```python
from build123d import *

# Parameters (mm, degrees)
SKETCH3_R            = 12.7
BOSS_EXTRUDE1_DEPTH  = 76.2
BOSS_EXTRUDE2_DEPTH  = 6.35
SKETCH6_W            = 63.5
SKETCH6_H            = 50.8
BOSS_EXTRUDE3_DEPTH  = 6.35
SKETCH9_W            = 50.8
SKETCH9_H            = 6.35
BOSS_EXTRUDE4_DEPTH  = 0.38862
SKETCH10_W           = 0.38862
SKETCH10_H           = 50.8
BOSS_EXTRUDE5_DEPTH  = 25.4
SKETCH11_W           = 50.8
SKETCH11_H           = 6.35
BOSS_EXTRUDE6_DEPTH  = 0.38862
SKETCH13_W           = 0.38862
SKETCH13_H           = 50.8
BOSS_EXTRUDE7_DEPTH  = 25.4
SKETCH14_W           = 0.38862
SKETCH14_H           = 50.8
BOSS_EXTRUDE8_DEPTH  = 10.8712
SKETCH15_W           = 50.8
SKETCH15_H           = 10.8712
BOSS_EXTRUDE9_DEPTH  = 25.76322
SKETCH16_W           = 0.38862
SKETCH16_H           = 50.8
BOSS_EXTRUDE10_DEPTH = 10.8712
SKETCH17_W           = 50.8
SKETCH17_H           = 10.8712
BOSS_EXTRUDE11_DEPTH = 25.76322


with BuildPart() as part:
    # Sketch3 → Boss-Extrude1 (new body)
    with BuildSketch(Plane.XY):
        with Locations(Location((0, 0, 0), (0, 0, 180))):
            Circle(SKETCH3_R)
    extrude(amount=BOSS_EXTRUDE1_DEPTH)

    # Sketch4 → Boss-Extrude2 (add)
    with BuildSketch(Plane(origin=(0, 0, 0), x_dir=(-1, 0, 0), z_dir=(0, 0, -1))):
        Polygon((0, 0), (19.05, 0), (19.05, 50.8), (-19.05, 50.8), (-19.05, 0), align=None)
    extrude(amount=-BOSS_EXTRUDE2_DEPTH)

    # Sketch6 → Boss-Extrude3 (add)
    with BuildSketch(Plane(origin=(0, 50.8, 0), x_dir=(1, 0, 0), z_dir=(0, 1, 0))):
        with Locations((1.04805825, -17.613482739)):
            Rectangle(SKETCH6_W, SKETCH6_H)
    extrude(amount=BOSS_EXTRUDE3_DEPTH)

    # Sketch9 → Boss-Extrude4 (add)
    with BuildSketch(Plane(origin=(32.79805825, 0, 0), x_dir=(0, 0, -1), z_dir=(1, 0, 0))):
        with Locations((-17.613482739, 53.975)):
            Rectangle(SKETCH9_W, SKETCH9_H)
    extrude(amount=BOSS_EXTRUDE4_DEPTH)

    # Sketch10 → Boss-Extrude5 (add)
    with BuildSketch(Plane(origin=(0, 57.15, 0), x_dir=(1, 0, 0), z_dir=(0, 1, 0))):
        with Locations((32.99236825, -17.613482739)):
            Rectangle(SKETCH10_W, SKETCH10_H)
    extrude(amount=BOSS_EXTRUDE5_DEPTH)

    # Sketch11 → Boss-Extrude6 (add)
    with BuildSketch(Plane.ZY.offset(30.70194175)):
        with Locations((17.613482739, 53.975)):
            Rectangle(SKETCH11_W, SKETCH11_H)
    extrude(amount=BOSS_EXTRUDE6_DEPTH)

    # Sketch13 → Boss-Extrude7 (add)
    with BuildSketch(Plane(origin=(0, 57.15, 0), x_dir=(1, 0, 0), z_dir=(0, 1, 0))):
        with Locations((-30.89625175, -17.613482739)):
            Rectangle(SKETCH13_W, SKETCH13_H)
    extrude(amount=BOSS_EXTRUDE7_DEPTH)

    # Sketch14 → Boss-Extrude8 (add)
    with BuildSketch(Plane(origin=(0, 82.55, 0), x_dir=(1, 0, 0), z_dir=(0, 1, 0))):
        with Locations((-30.89625175, -17.613482739)):
            Rectangle(SKETCH14_W, SKETCH14_H)
    extrude(amount=BOSS_EXTRUDE8_DEPTH)

    # Sketch15 → Boss-Extrude9 (add)
    with BuildSketch(Plane(origin=(-30.70194175, 0, 0), x_dir=(0, 0, -1), z_dir=(1, 0, 0))):
        with Locations((-17.613482739, 87.9856)):
            Rectangle(SKETCH15_W, SKETCH15_H)
    extrude(amount=BOSS_EXTRUDE9_DEPTH)

    # Sketch16 → Boss-Extrude10 (add)
    with BuildSketch(Plane(origin=(0, 82.55, 0), x_dir=(1, 0, 0), z_dir=(0, 1, 0))):
        with Locations((32.99236825, -17.613482739)):
            Rectangle(SKETCH16_W, SKETCH16_H)
    extrude(amount=BOSS_EXTRUDE10_DEPTH)

    # Sketch17 → Boss-Extrude11 (add)
    with BuildSketch(Plane.ZY.offset(-32.79805825)):
        with Locations((17.613482739, 87.9856)):
            Rectangle(SKETCH17_W, SKETCH17_H)
    extrude(amount=BOSS_EXTRUDE11_DEPTH)


solid = part.part
```
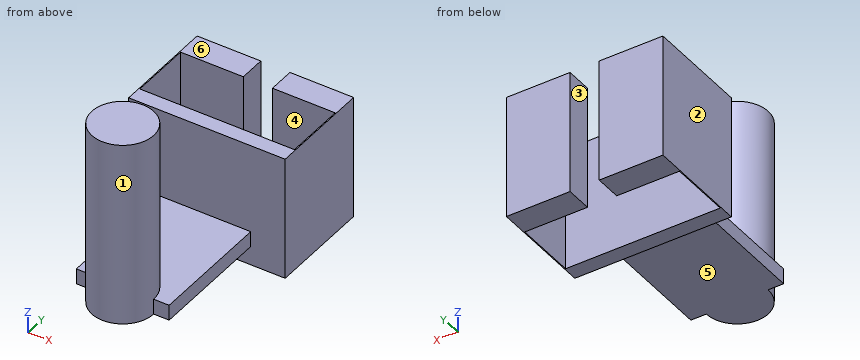
Geometry check sheet. Reference: the model listing, model coordinates, mm. Face numbers are marked on the shaded views. A direction names the side the tool comes from. Round coordinates to 2 decimals unless told otherwise and drop trailing zeros. Loops run counter-clockwise (first coordinate to the right, second up) from the corner with the lowest first, then second, coordinate; pieces in that order, holes last. Notation, with made-up numbers: (-39.5, 23.25) -> (15.5, 23.25) arc R20 cw to (15.5, 32.25) -> close; hole circle Ø2 at (70.5, -1). An arc over 180 degrees is marked (long way). Use a Markdown table: item, result.
(1) Sectioned sample at D-D (z = 1.5). Enter the section's corners in (x, y).
Calculated:
| item | result |
|---|---|
| outline | (-31.09, 50.8) -> (-19.05, 50.8) -> (-19.05, 0) -> (-12.7, 0) arc R12.7 ccw to (12.7, 0) -> (19.05, 0) -> (19.05, 50.8) -> (33.19, 50.8) -> (33.19, 93.42) -> (7.03, 93.42) -> (7.03, 82.55) -> (32.8, 82.55) -> (32.8, 57.15) -> (-30.7, 57.15) -> (-30.7, 82.55) -> (-4.94, 82.55) -> (-4.94, 93.42) -> (-31.09, 93.42) -> close |
(2) Sectioned sample at A-A (z = 35). Enter the section's corners in (x, y), then the cut area to 3 significant figures.
Calculated:
| item | result |
|---|---|
| outline | (-31.09, 50.8) -> (33.19, 50.8) -> (33.19, 93.42) -> (7.03, 93.42) -> (7.03, 82.55) -> (32.8, 82.55) -> (32.8, 57.15) -> (-30.7, 57.15) -> (-30.7, 82.55) -> (-4.94, 82.55) -> (-4.94, 93.42) -> (-31.09, 93.42) -> close; circle Ø25.4 at (0, 0) |
| area | 1,500 mm² |
(3) Sectioned sample at B-B (x = -8.5). Enter the section's corners in (y, z).
Calculated:
| item | result |
|---|---|
| outline | (-9.44, 0) -> (50.8, 0) -> (50.8, -7.79) -> (57.15, -7.79) -> (57.15, 43.01) -> (50.8, 43.01) -> (50.8, 6.35) -> (9.44, 6.35) -> (9.44, 76.2) -> (-9.44, 76.2) -> close; (82.55, -7.79) -> (93.42, -7.79) -> (93.42, 43.01) -> (82.55, 43.01) -> close |
(4) Sectioned sample at C-C (y = 62.5). Enter the section's corners in (x, z), then the cut area to 3 significant figures.
Calculated:
| item | result |
|---|---|
| outline | (-31.09, -7.79) -> (-30.7, -7.79) -> (-30.7, 43.01) -> (-31.09, 43.01) -> close; (32.8, -7.79) -> (33.19, -7.79) -> (33.19, 43.01) -> (32.8, 43.01) -> close |
| area | 39.5 mm² |
(5) Mould release check, pull along X, two halves, no side actions. Record for the marked faces 1, 2 and 3: released by +X, released by -X, zero draft, split by the parting line, or undercut.
Calculated:
| item | result |
|---|---|
| face 1 | split by the parting line |
| face 2 | released by -X |
| face 3 | undercut |
(6) Go/stop test with flat-tipped pins: P1, Ø1.5, axis at x = 4.5, z = 41, coming from the +Y side; P2, Ø19, axis at x = -7, y = 36.5, coming from the +Z side; P3, Ø5, axis at y = 37.5, z = 2.5, coming from the +X side; P4, Ø1, axis at x = -14, z = 65, coming from the +Y side. Record where each tip stops, or that it passes through.
Calculated:
| item | result |
|---|---|
| P1 | y = 57.15 |
| P2 | z = 6.35 |
| P3 | x = 19.05 |
| P4 | through |
(7) Set-up check for the marked faces 4, 5 and 6: record each of +Z, -Z, +X, -X, +Y, -Y from which the full face is reachable in a straight line by a thin tool's end or side.
Calculated:
| item | result |
|---|---|
| face 4 | +Z, -Z |
| face 5 | -Z, +X, -X, -Y |
| face 6 | +Z, +X, -X, +Y |
(8) Scan lines: probe 1 along Y at (x, z) = (-6, -4); probe 2 along Y at (x, z) = (11.5, 20); probe 3 along X at (y, z) = (72.5, -2.5). Record each from-to range of solid material in increasing order.
Calculated:
| item | result |
|---|---|
| probe 1 | 50.8 to 57.15, 82.55 to 93.42 |
| probe 2 | -5.39 to 5.39, 50.8 to 57.15, 82.55 to 93.42 |
| probe 3 | -31.09 to -30.7, 32.8 to 33.19 |
